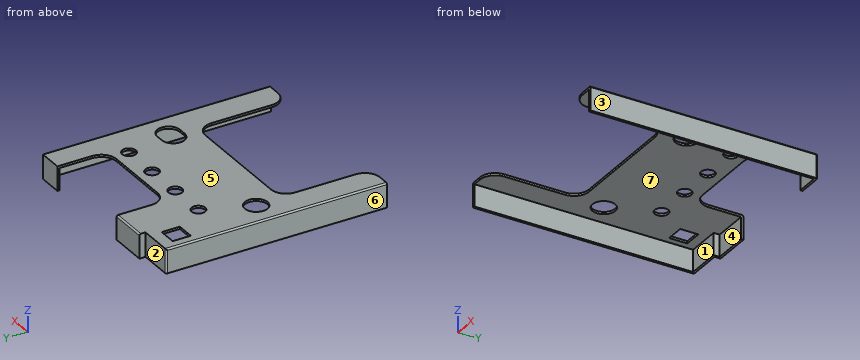
from build123d import *

# Parameters (mm, degrees)
F0_R     = 0.75
F0_R_2   = 0.45
F0_W     = 1.2
F0_H     = 1.2
F1_DEPTH = 0.15
F2_W     = 1.5
F2_H     = 0.15
F2_W_2   = 0.15
F2_H_2   = 14.45
F3_DEPTH = 1.45
F4_R     = 1
F5_R     = 0.1


with BuildPart() as f1:
    # F0 (on Top) → F1 (new body)
    with BuildSketch(Plane.XY):
        Polygon((0, 14.6), (0, 0), (1.77, 0), (1.77, 6), (10.97, 6), (10.97, 0), (12.9, 0), (12.9, 15), (11.25, 15), (11.25, 11.7), (4.75, 11.7), (4.75, 15), (2.25, 15), (2.25, 14.6), align=None)
        with Locations((1.65, 7.65)):
            Circle(F0_R, mode=Mode.SUBTRACT)
        with Locations((2.92, 10.7)):
            Circle(F0_R_2, mode=Mode.SUBTRACT)
        with Locations((5.46, 10.7)):
            Circle(F0_R_2, mode=Mode.SUBTRACT)
        with Locations((1.2, 13.2)):
            Rectangle(F0_W, F0_H, mode=Mode.SUBTRACT)
        with Locations((8, 10.7)):
            Circle(F0_R_2, mode=Mode.SUBTRACT)
        with BuildLine():
            ThreePointArc((11.25, 8.4), (12, 7.65), (11.25, 6.9))
            Line((11.25, 6.9), (10.75, 6.9))
            ThreePointArc((10.75, 6.9), (10, 7.65), (10.75, 8.4))
            Line((10.75, 8.4), (11.25, 8.4))
        make_face(mode=Mode.SUBTRACT)
        with Locations((10.54, 10.7)):
            Circle(F0_R_2, mode=Mode.SUBTRACT)
    extrude(amount=F1_DEPTH)

    # F2 (on face) → F3 (join)
    with BuildSketch(Plane(origin=(0, 0, 0), x_dir=(1, 0, 0), z_dir=(0, 0, -1))):
        Polygon((12.9, -15), (12.9, 0), (12.75, 0), (12.75, -14.85), (12.75, -15), align=None)
        with Locations((12, -14.925)):
            Rectangle(F2_W, F2_H)
        Polygon((4.75, -15), (4.75, -14.85), (2.4, -14.85), (2.25, -14.85), (2.25, -15), align=None)
        Polygon((2.25, -14.85), (2.4, -14.85), (2.4, -14.45), (2.25, -14.45), (2.25, -14.6), align=None)
        Polygon((2.25, -14.45), (0.15, -14.45), (0, -14.45), (0, -14.6), (2.25, -14.6), align=None)
        with Locations((0.075, -7.225)):
            Rectangle(F2_W_2, F2_H_2)
    extrude(amount=F3_DEPTH)

    # F4
    f4_edges = [f1.edges().sort_by_distance(p)[0] for p in [
        (1.77, 6, 0.075),
        (1.77, 0, 0.075),
        (10.97, 6, 0.075),
        (10.97, 0, 0.075),
        (4.75, 11.7, 0.075),
        (11.25, 11.7, 0.075),
    ]]
    fillet(f4_edges, radius=F4_R)

    # F5
    f5_edges = [f1.edges().sort_by_distance(p)[0] for p in [
        (12.9, 7.5, 0.15),
        (0, 7.3, 0.15),
        (3.5, 15, 0.15),
        (0, 14.6, -0.65),
        (12.9, 15, -0.65),
    ]]
    fillet(f5_edges, radius=F5_R)


solid = f1.part
Design review of the part built by this model. Coordinates are the model's own, in mm. Face numbers are marked on the shaded views. A direction names the side the tool comes from. Round coordinates to 2 decimals unless told otherwise and drop trailing zeros. Order: outer loops, then holes, each group sorted by start corner. A loop starts at its lowest first (then second) coordinate and runs counter-clockwise, first axis right, second up.
1) Clearance check with a flat-ended pin moving along its axis: pin 1 Ø6 at (x, y) = (8.5, 12.5) entering from -Z. State where the tip first meets the part, or that it passes through.
The answers:
pin 1: stops at z = 0
2) Consider section B-B (x = 8). State the section outline as (y, z) points.
The answers:
outline: (6, 0) - (10.25, 0) - (10.25, 0.15) - (6, 0.15) - close; (11.15, 0) - (11.7, 0) - (11.7, 0.15) - (11.15, 0.15) - close
3) For L1, parallel to X at y = 4.75, z = -1.3; L2, parallel to Y at x = 10.54, z = 0.1; L3, parallel to Y at x = 1.65, z = 0.1, list the stretches that pass through material, from the lowest coordinate up.
The answers:
L1: x = 0 to 0.15, 12.75 to 12.9
L2: y = 5.82 to 6.93, 8.37 to 10.25, 11.15 to 11.74
L3: y = 0.53 to 6.9, 8.4 to 12.6, 13.8 to 14.6
4) Consider section C-C (y = 7.65). State the section outline as (x, z) points, plus the area to 3 significant figures.
The answers:
outline: (0, -1.45) - (0.15, -1.45) - (0.15, 0) - (0.9, 0) - (0.9, 0.15) - (0.1, 0.15) arc R0.1 ccw to (0, 0.05) - close; (2.4, 0) - (10, 0) - (10, 0.15) - (2.4, 0.15) - close; (12, 0) - (12.75, 0) - (12.75, -1.45) - (12.9, -1.45) - (12.9, 0.05) arc R0.1 ccw to (12.8, 0.15) - (12, 0.15) - close
area: 1.84 mm2
5) Consider section D-D (y = 12.25). State the section outline as (x, z) points, plus the area to 3 significant figures.
The answers:
outline: (0, -1.45) - (0.15, -1.45) - (0.15, 0) - (4.86, 0) - (4.86, 0.15) - (0.1, 0.15) arc R0.1 ccw to (0, 0.05) - close; (11.14, 0) - (12.75, 0) - (12.75, -1.45) - (12.9, -1.45) - (12.9, 0.05) arc R0.1 ccw to (12.8, 0.15) - (11.14, 0.15) - close
area: 1.42 mm2
6) Draft analysis for pull direction X (two halves, no side actions). For the marked faces 4, 5, 6 and 7, state which applies: released by +X, released by -X, zero draft, split by the parting line, or undercut.
The answers:
face 4: undercut
face 5: zero draft
face 6: released by -X
face 7: undercut
7) Machinability: for the marked faces 1, 2 and 3, which of the approach directions +Z, -Z, +X, -X, +Y, -Y give a long, thin tool a straight path to every point of the face, cutting with its end or side? Answer none if there is none.
The answers:
face 1: -Z, -Y
face 2: +Z, -Z, -X, +Y
face 3: +Z, -Z, +X, +Y, -Y
8) Consider section A-A (z = -0.8). State the section outline as (x, y) points.
The answers:
outline: (0, 0) - (0.15, 0) - (0.15, 14.45) - (2.4, 14.45) - (2.4, 14.85) - (4.75, 14.85) - (4.75, 15) - (2.25, 15) - (2.25, 14.6) - (0.1, 14.6) arc R0.1 ccw to (0, 14.5) - close; (11.25, 14.85) - (12.75, 14.85) - (12.75, 0) - (12.9, 0) - (12.9, 14.9) arc R0.1 ccw to (12.8, 15) - (11.25, 15) - close
